Study the drawing (mm; zero at the part's minimum x, y, z) and answer. A direction names the side the tool comes from. Give positions to 0.01 mm unless a question says otherwise; leave off trailing zeros. Loops run counter-clockwise (first coordinate to the right, second up) from the corner with the lowest first, then second, coordinate; pieces in that order, holes last. Notation, with made-up numbers: (40, 41.25) - (74, 41.25) arc R17 cw to (74, 50.25) - close; hole circle Ø7 at (79, 2). An arc over 180 degrees is marked (long way). Write item = value, one per line. Start each with the question number.
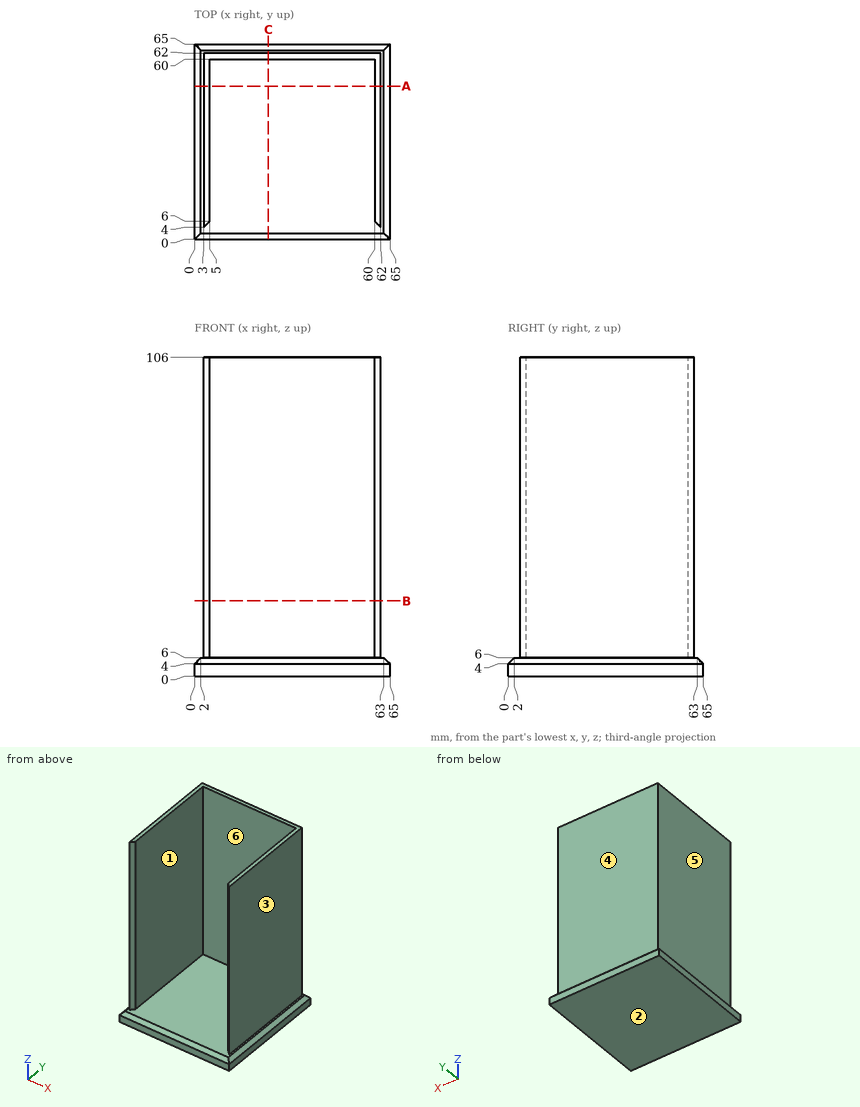
1. Given P1, Ø4, axis at x = 13, z = 24.5, coming from the -Y side; P2, Ø5, axis at y = 31.5, z = 75.5, coming from the -X side; P3, Ø2, axis at x = 36, z = 77, coming from the +Y side, each flat-ended and moving along its own axis, determine where each tip first touches the part or whether it passes through.
2. A cutting plane is placed at A-A on y = 51. Give the vertices of the cut face in (x, z), and give its area (3 significant figures).
3. A tool of negligible diameter and unlimited length cuts with its end or side. For the marked faces 1, 2 and 3, from which of +Z, -Z, +X, -X, +Y, -Y can it reach the whole face along a straight path? Write none if from no direction.
4. A cutting plane is placed at B-B on z = 25. Give the vertices of the cut face in (x, y), and give its area (3 significant figures).
5. For a pull along X with two mould halves and no side action, classify the marked faces 4, 5 and 6 as released by +X, released by -X, zero draft, split by the parting line, or undercut.
6. A cutting plane is placed at C-C on x = 24.5. Give the vertices of the cut face in (y, z), and give its area (3 significant figures).
7. Consider line 1 along X through (y, z) = (59, 29); line 2 along Z through (x, y) = (31, 16.5); line 3 along Y through (x, z) = (11, 76). Determine where each line is inside the solid, lowest interval first. Write a range as [from, to].
Reply:
q1.P1 = 60
q1.P2 = 3
q1.P3 = 62
q2.outline = (0, 0) - (65, 0) - (65, 4) - (63, 6) - (62, 6) - (62, 106) - (60, 106) - (60, 6) - (5, 6) - (5, 106) - (3, 106) - (3, 6) - (2, 6) - (0, 4) - close
q2.area = 786 mm^2
q3.face_1 = +Z, -Y
q3.face_2 = -Z, +X, -X, +Y, -Y
q3.face_3 = +Z, +X, +Y, -Y
q4.outline = (3, 4) - (5, 6) - (5, 60) - (60, 60) - (60, 6) - (62, 4) - (62, 62) - (3, 62) - close
q4.area = 338 mm^2
q5.face_4 = zero draft
q5.face_5 = released by -X
q5.face_6 = undercut
q6.outline = (0, 0) - (65, 0) - (65, 4) - (63, 6) - (62, 6) - (62, 106) - (60, 106) - (60, 6) - (2, 6) - (0, 4) - close
q6.area = 586 mm^2
q7.line_1 = [3, 5], [60, 62]
q7.line_2 = [0, 6]
q7.line_3 = [60, 62]
